from build123d import *

# Parameters (mm, degrees)
SKETCH1_W           = 38
SKETCH1_H           = 22
BOSS_EXTRUDE1_DEPTH = 33
SKETCH2_W           = 35
SKETCH2_H           = 17
CUT_EXTRUDE1_DEPTH  = 28
SKETCH3_W           = 6
SKETCH3_H           = 17
BOSS_EXTRUDE2_DEPTH = 17.5
SKETCH4_W           = 42
SKETCH4_H           = 26
SKETCH4_W_2         = 38
SKETCH4_H_2         = 22
EXTRUDE_THIN2_DEPTH = 1.4
SKETCH5_R           = 1
CUT_EXTRUDE2_DEPTH  = 3
SKETCH6_R           = 1
CUT_EXTRUDE3_DEPTH  = 3
SKETCH7_W           = 9.4
SKETCH7_H           = 4.5
CUT_EXTRUDE4_DEPTH  = 10
SKETCH8_W           = 20
SKETCH8_H           = 10
CUT_EXTRUDE5_DEPTH  = 3.5
SKETCH9_R           = 3.7
SKETCH9_R_2         = 1
CUT_EXTRUDE6_DEPTH  = 47.845174865
FILLET1_R           = 4
FILLET2_R           = 3
FILLET3_R           = 4


with BuildPart() as part:
    # Sketch1 → Boss-Extrude1 (new body)
    with BuildSketch(Plane(origin=(0, 0, 0), x_dir=(1, 0, 0), z_dir=(0, 1, 0))):
        with Locations((8.6, -5.057142857)):
            Rectangle(SKETCH1_W, SKETCH1_H)
    extrude(amount=BOSS_EXTRUDE1_DEPTH)

    # Sketch2 → Cut-Extrude1 (cut)
    with BuildSketch(Plane(origin=(0, 33, 0), x_dir=(1, 0, 0), z_dir=(0, 1, 0))):
        with Locations((8.5, -3.957142857)):
            Rectangle(SKETCH2_W, SKETCH2_H)
    extrude(amount=-CUT_EXTRUDE1_DEPTH, mode=Mode.SUBTRACT)

    # Sketch3 → Boss-Extrude2 (add)
    with BuildSketch(Plane(origin=(0, 5, 0), x_dir=(1, 0, 0), z_dir=(0, 1, 0))):
        with Locations((-6, -3.957142857)):
            Rectangle(SKETCH3_W, SKETCH3_H)
        with Locations((23, -3.957142857)):
            Rectangle(SKETCH3_W, SKETCH3_H)
    extrude(amount=BOSS_EXTRUDE2_DEPTH)

    # Sketch4 → Extrude-Thin2 (add)
    with BuildSketch(Plane(origin=(0, 33, 0), x_dir=(1, 0, 0), z_dir=(0, 1, 0))):
        with Locations((8.6, -5.057142857)):
            Rectangle(SKETCH4_W, SKETCH4_H)
        with Locations((8.6, -5.057142857)):
            Rectangle(SKETCH4_W_2, SKETCH4_H_2, mode=Mode.SUBTRACT)
    extrude(amount=-EXTRUDE_THIN2_DEPTH)

    # Sketch5 → Cut-Extrude2 (cut)
    with BuildSketch(Plane(origin=(0, 22.5, 0), x_dir=(1, 0, 0), z_dir=(0, 1, 0))):
        with Locations(Location((-5.5, -3.892148731, 0), (0, 0, 270))):
            Circle(SKETCH5_R)
    extrude(amount=-CUT_EXTRUDE2_DEPTH, mode=Mode.SUBTRACT)

    # Sketch6 → Cut-Extrude3 (cut)
    with BuildSketch(Plane(origin=(0, 22.5, 0), x_dir=(1, 0, 0), z_dir=(0, 1, 0))):
        with Locations(Location((22.953148274, -4.115727136, 0), (0, 0, 270))):
            Circle(SKETCH6_R)
    extrude(amount=-CUT_EXTRUDE3_DEPTH, mode=Mode.SUBTRACT)

    # Sketch7 → Cut-Extrude4 (cut)
    with BuildSketch(Plane(origin=(-3, 0, 0), x_dir=(0, 0, -1), z_dir=(1, 0, 0))):
        with Locations((-3.757142857, 6.291369126)):
            Rectangle(SKETCH7_W, SKETCH7_H)
    extrude(amount=-CUT_EXTRUDE4_DEPTH, mode=Mode.SUBTRACT)

    # Sketch8 → Cut-Extrude5 (cut)
    with BuildSketch(Plane(origin=(0, 5, 0), x_dir=(1, 0, 0), z_dir=(0, 1, 0))):
        with Locations((8.592117784, -3.72787339)):
            Rectangle(SKETCH8_W, SKETCH8_H)
    extrude(amount=-CUT_EXTRUDE5_DEPTH, mode=Mode.SUBTRACT)

    # Sketch9 → Cut-Extrude6 (cut, through all)
    with BuildSketch(Plane(origin=(0, 1.5, 0), x_dir=(1, 0, 0), z_dir=(0, 1, 0))):
        with Locations(Location((8.808284604, -3.634888569, 0), (0, 0, 270))):
            Circle(SKETCH9_R)
        with Locations(Location((1.608284604, -3.634888569, 0), (0, 0, 270))):
            Circle(SKETCH9_R_2)
        with Locations(Location((16.008284604, -3.634888569, 0), (0, 0, 270))):
            Circle(SKETCH9_R_2)
    extrude(amount=-CUT_EXTRUDE6_DEPTH, mode=Mode.SUBTRACT)

    # Fillet1
    fillet1_edges = [part.edges().sort_by_distance(p)[0] for p in [
        (-1.407882216, 3.25, 8.72787339),
        (-1.407882216, 3.25, -1.27212661),
        (18.592117784, 3.25, -1.27212661),
        (18.592117784, 3.25, 8.72787339),
    ]]
    fillet(fillet1_edges, radius=FILLET1_R)

    # Fillet2
    fillet2_edges = [part.edges().sort_by_distance(p)[0] for p in [
        (-3, 8.541369126, 3.757142857),
    ]]
    fillet(fillet2_edges, radius=FILLET2_R)

    # Fillet3
    # the kernel refuses this fillet: 4 mm, written as the material it adds along each edge
    with BuildSketch(Plane(origin=(-10.4, 31.6, 16.057142857), x_dir=(-1, 0, 0), z_dir=(0, 0, -1)), Plane(origin=(27.6, 31.6, -5.942857143), x_dir=(1, 0, 0), z_dir=(0, 0, 1))) as fillet3_piece_1:
        with BuildLine():
            CenterArc((4, -3.464101615), FILLET3_R, 120, 60)
            Line((0, -3.464101615), (-0.08, -3.464101615))
            Line((-0.08, -3.464101615), (-0.08, 0))
            Line((-0.08, 0), (0, 0.08))
            ThreePointArc((0, 0.08), (1, 0.08), (1.96, 0.069282032))
            Line((1.96, 0.069282032), (2, 0))
        make_face()
    extrude(amount=22)


solid = part.part
Geometry: final body of the model. Coordinates: model frame, mm. A direction names the side the tool comes from. Coordinates: 2 decimals unless noted, no trailing zeros. Order: outer loops, then holes, each group sorted by start corner. A loop starts at its lowest first (then second) coordinate and runs counter-clockwise, first axis right, second up. Notation, with made-up numbers: M 83,-30 L 125,-30 A29 cw 125,6 Z; hole C 28,36.5 d6. An arc over 180 degrees is marked long. One line per question, with ' | ' between items. Start each with the question number.
Item 1: Cut plane B-B, the plane y = 3. Return the cut outline in (x, z), then the cut area to 3 significant figures.
Item 2: Cut plane D-D, the plane x = -5.5. Return the cut outline in (y, z).
Item 3: Ray query, probe 1 along Z at (x, y) = (-4, 29.5); probe 2 along X at (y, z) = (15.5, 10.5); probe 3 along X at (y, z) = (26.5, -1.25). Return the intervals inside material, ascending. Write a range as [from, to].
Item 4: Cut plane A-A, the plane x = 7. Return the cut outline in (y, z), then the cut area to 3 significant figures.
Item 5: Draft query along Z for faces 6 (the flat face through (18.592, 3, 4)), 7 (the flat face through (-10.4, 14, 5)). Return one class per face: released by +Z, released by -Z, zero draft, split by the parting line, or undercut.
Item 6: Cut plane C-C, the plane z = -3. Return the cut outline in (x, y).
Item 7: Set-up query: faces 1 (the cylindrical face through (1.91, 0.76, 4.59)), 2 (the flat face through (8, 19, -4.543)), 3 (the cylindrical face through (-3.9, 9.4, 3.7)), 4 (the flat face through (-7, 4.041, 4)), 5 (the flat face through (8, 31.6, -7)). Return all of +Z, -Z, +X, -X, +Y, -Y with unobstructed straight access to the full face (end or side cutting, diameter ignored); none if empty.
Item 8: Pin query (flat end, axial travel): pin 1 Ø3 at (y, z) = (15.5, 7) entering from +X; pin 2 Ø13.5 at (x, z) = (8, 4) entering from +Y; pin 3 Ø0.6 at (x, z) = (22.5, 4) entering from +Y. Return the tip coordinate at first contact, or that it passes through.
A:
1) outline: M -10.4,-5.94 L 27.6,-5.94 L 27.6,16.06 L -10.4,16.06 Z; hole M -1.41,2.73 A4 ccw 2.59,-1.27 L 14.59,-1.27 A4 ccw 18.59,2.73 L 18.59,4.73 A4 ccw 14.59,8.73 L 2.59,8.73 A4 ccw -1.41,4.73 Z | area: 650 mm2
2) outline: M 0,-5.94 L 31.6,-5.94 L 31.6,-7.94 L 33,-7.94 L 33,-4.54 L 22.5,-4.54 L 22.5,2.89 L 19.5,2.89 L 19.5,4.89 L 22.5,4.89 L 22.5,12.46 L 33,12.46 L 33,18.06 L 31.6,18.06 L 31.6,16.06 L 0,16.06 Z; hole M 4.04,-0.94 L 8.58,-0.94 L 8.58,8.46 L 4.04,8.46 Z
3) probe 1: z = [-5.94, -4.54], [12.46, 16.06] | probe 2: x = [-10.4, -3], [20, 27.6] | probe 3: x = [-10.4, -9], [26, 27.6]
4) outline: M 0,-5.94 L 31.6,-5.94 L 31.6,-7.94 L 33,-7.94 L 33,-4.54 L 5,-4.54 L 5,-1.27 L 1.5,-1.27 L 1.5,0.41 L 0,0.41 Z; M 0,6.86 L 1.5,6.86 L 1.5,8.73 L 5,8.73 L 5,12.46 L 33,12.46 L 33,18.06 L 31.6,18.06 L 31.6,16.06 L 0,16.06 Z | area: 211 mm2
5) face 6: undercut | face 7: zero draft
6) outline: M -12.4,31.6 A4 cw -10.4,28.14 L -10.4,0 L 27.6,0 L 27.6,28.14 A4 cw 29.6,31.6 L 29.6,33 L 26,33 L 26,22.5 L 20,22.5 L 20,5 L -3,5 L -3,22.5 L -9,22.5 L -9,33 L -12.4,33 Z
7) face 1: +Y, -Y | face 2: +Y | face 3: none | face 4: -X | face 5: -Z, +X, -X, -Y
8) pin 1: stops at x = 27.6 | pin 2: stops at y = 5 | pin 3: stops at y = 19.5
